from build123d import *

# Parameters (mm, degrees)
ESQUISSE3_R          = 7.5
ESQUISSE3_R_2        = 2.8
BOSS_EXTRU_1_DEPTH   = 2
BOSS_EXTRU_1_2_DEPTH = 2
BOSS_EXTRU_1_3_DEPTH = 2
BOSS_EXTRU_1_4_DEPTH = 2
ESQUISSE4_R          = 7.5
ESQUISSE4_R_2        = 1.7
BOSS_EXTRU_2_DEPTH   = 3
BOSS_EXTRU_3_DEPTH   = 5
BOSS_EXTRU_4_START   = -2
ESQUISSE6_W          = 123.2
ESQUISSE6_H          = 7
BOSS_EXTRU_4_DEPTH   = 10


with BuildPart() as part:
    # Esquisse3 → Boss.-Extru.1 (new body)
    with BuildSketch(Plane(origin=(0, 0, 0), x_dir=(1, 0, 0), z_dir=(0, 0.342020143, 0.939692621))):
        with Locations((-54.1, 26.6)):
            Circle(ESQUISSE3_R)
        with Locations((-54.1, 26.6)):
            Circle(ESQUISSE3_R_2, mode=Mode.SUBTRACT)
    extrude(amount=BOSS_EXTRU_1_DEPTH)



with BuildPart() as body_2:
    # Esquisse3 → Boss.-Extru.1 2 (new body)
    with BuildSketch(Plane(origin=(0, 0, 0), x_dir=(1, 0, 0), z_dir=(0, 0.342020143, 0.939692621))):
        with Locations((54.1, 26.6)):
            Circle(ESQUISSE3_R)
        with Locations((54.1, 26.6)):
            Circle(ESQUISSE3_R_2, mode=Mode.SUBTRACT)
    extrude(amount=BOSS_EXTRU_1_2_DEPTH)


with BuildPart() as body_3:
    # Esquisse3 → Boss.-Extru.1 3 (new body)
    with BuildSketch(Plane(origin=(0, 0, 0), x_dir=(1, 0, 0), z_dir=(0, 0.342020143, 0.939692621))):
        with Locations((54.1, -26.6)):
            Circle(ESQUISSE3_R)
        with Locations((54.1, -26.6)):
            Circle(ESQUISSE3_R_2, mode=Mode.SUBTRACT)
    extrude(amount=BOSS_EXTRU_1_3_DEPTH)


with BuildPart() as body_4:
    # Esquisse3 → Boss.-Extru.1 4 (new body)
    with BuildSketch(Plane(origin=(0, 0, 0), x_dir=(1, 0, 0), z_dir=(0, 0.342020143, 0.939692621))):
        with Locations((-54.1, -26.6)):
            Circle(ESQUISSE3_R)
        with Locations((-54.1, -26.6)):
            Circle(ESQUISSE3_R_2, mode=Mode.SUBTRACT)
    extrude(amount=BOSS_EXTRU_1_4_DEPTH)


with BuildPart() as part_1:
    add(part.part)

    add(body_2.part)  # Boss.-Extru.2 merges body 2

    add(body_3.part)  # Boss.-Extru.2 merges body 3

    add(body_4.part)  # Boss.-Extru.2 merges body 4
    # Esquisse4 → Boss.-Extru.2 (add)
    with BuildSketch(Plane(origin=(0, 0, 0), x_dir=(-1, 0, 0), z_dir=(0, -0.342020143, -0.939692621))):
        with Locations((-54.1, 26.6)):
            Circle(ESQUISSE4_R)
        with Locations((-54.1, 26.6)):
            Circle(ESQUISSE4_R_2, mode=Mode.SUBTRACT)
        with Locations((54.1, 26.6)):
            Circle(ESQUISSE4_R)
        with Locations((54.1, 26.6)):
            Circle(ESQUISSE4_R_2, mode=Mode.SUBTRACT)
        with Locations((54.1, -26.6)):
            Circle(ESQUISSE4_R)
        with Locations((54.1, -26.6)):
            Circle(ESQUISSE4_R_2, mode=Mode.SUBTRACT)
        with Locations((-54.1, -26.6)):
            Circle(ESQUISSE4_R)
        with Locations((-54.1, -26.6)):
            Circle(ESQUISSE4_R_2, mode=Mode.SUBTRACT)
    extrude(amount=BOSS_EXTRU_2_DEPTH)

    # Esquisse5 → Boss.-Extru.3 (add)
    with BuildSketch(Plane(origin=(0, -1.02606043, -2.819077862), x_dir=(-1, 0, 0), z_dir=(0, -0.342020143, -0.939692621))):
        with BuildLine():
            Line((-61.6, 26.6), (-61.6, -26.6))
            ThreePointArc((-61.6, -26.6), (-54.1, -19.1), (-46.6, -26.6))
            Line((-46.6, -26.6), (-46.6, 26.6))
            ThreePointArc((-46.6, 26.6), (-54.1, 19.1), (-61.6, 26.6))
        make_face()
        with BuildLine():
            Line((61.6, 26.6), (61.6, -26.6))
            ThreePointArc((61.6, -26.6), (54.1, -19.1), (46.6, -26.6))
            Line((46.6, -26.6), (46.6, 26.6))
            ThreePointArc((46.6, 26.6), (54.1, 19.1), (61.6, 26.6))
        make_face()
    extrude(amount=-BOSS_EXTRU_3_DEPTH)

    # Esquisse6 → Boss.-Extru.4 (add)
    with BuildSketch(Plane(origin=(0, 0.684040287, 1.879385242), x_dir=(1, 0, 0), z_dir=(0, 0.342020143, 0.939692621)).offset(BOSS_EXTRU_4_START)):
        with Locations((0, 34.85)):
            Rectangle(ESQUISSE6_W, ESQUISSE6_H)
    extrude(amount=BOSS_EXTRU_4_DEPTH)


solid = part_1.part
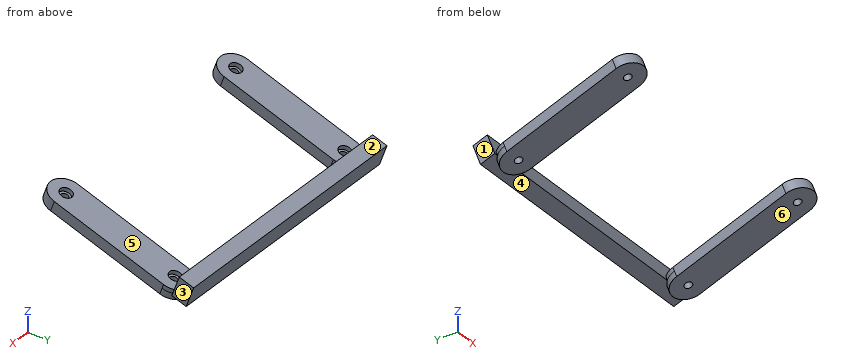
Source: CAD feature listing. Evaluate the final solid. Frame: model axes, mm. Face numbers are marked on the shaded views. A direction names the side the tool comes from. Give positions to 0.01 mm unless a question says otherwise; leave off trailing zeros. Order: outer loops, then holes, each group sorted by start corner. A loop starts at its lowest first (then second) coordinate and runs counter-clockwise, first axis right, second up. Notation, with made-up numbers: (81, 82) -> (105, 82) arc R19 cw to (105, 87) -> close; hole circle Ø9 at (45, 23.25). An arc over 180 degrees is marked (long way). Use a Markdown table: item, result.
1) Reachability of the marked faces 5 and 6 from +Z, -Z, +X, -X, +Y, -Y: full face, straight path, thin tool, end or side. Return the list, or none.
Answer list:
| item | result |
|---|---|
| face 5 | +Z, +X, -X |
| face 6 | -Z, +X, -X, -Y |
2) Section query B-B, the plane x = -41. Return the cut outline in (y, z).
Answer list:
| item | result |
|---|---|
| outline | (29.46, -10.72) -> (36.04, -13.12) -> (39.46, -3.72) -> (32.88, -1.33) -> close |
3) Ray query, line 1 along X through (y, z) = (21, -7.5); line 2 along Z through (x, y) = (51, 6); line 3 along Z through (x, y) = (-52, 4). Return the intervals inside material, ascending. Write a range as [from, to].
Answer list:
| item | result |
|---|---|
| line 1 | [-61.6, -46.6], [46.6, 61.6] |
| line 2 | [-5.38, -0.06] |
| line 3 | [-4.65, 0.67] |
4) Mould query, pull axis X, two halves, no side actions, for the marked faces 1, 2, 3 and 4. Classes: +X half, -X half, draft (parallel to the pull), parting line (faces both ways), or undercut.
Answer list:
| item | result |
|---|---|
| face 1 | -X half |
| face 2 | draft |
| face 3 | +X half |
| face 4 | undercut |
5) Section query A-A, the plane y = 12. Return the cut outline in (x, z).
Answer list:
| item | result |
|---|---|
| outline | (-61.6, -7.56) -> (-46.6, -7.56) -> (-46.6, -2.24) -> (-61.6, -2.24) -> close; (46.6, -7.56) -> (61.6, -7.56) -> (61.6, -2.24) -> (46.6, -2.24) -> close |
6) Contact query for flat-ended pins moving along their axis: P1, Ø4, axis at y = 0.5, z = -4, coming from the +X side; P2, Ø3, axis at x = 17.5, z = -11, coming from the +Y side; P3, Ø8, axis at y = -21, z = -2, coming from the -X side; P4, Ø10, axis at x = -44, z = -8, coming from the +Y side. Output: stop coordinate, or through.
Answer list:
| item | result |
|---|---|
| P1 | x = 61.6 |
| P2 | y = 37.35 |
| P3 | through |
| P4 | y = 39.46 |
